Could you check a few things on this model? Use its own coordinates, in mm. A direction names the side the tool comes from. Coordinates: 2 decimals unless noted, no trailing zeros. Loops run counter-clockwise (first coordinate to the right, second up) from the corner with the lowest first, then second, coordinate; pieces in that order, holes last.
1) If I drill on line 1 along Y through (x, z) = (40, -0.25) (3 decimals); line 2 along Y through (x, z) = (50.8, -11.25), over which ranges is the centre line in solid material (lowest first)?
2) Imagine slicing it at A-A on y = 0. Please give me the cut outline in (x, z) (1 decimal).
3) For faces 4 (the face through (-1, 9.525, 0)), 5 (the face through (-1, 0, 12.7)), which set-ups out of +Z, -Z, +X, -X, +Y, -Y let a thin tool reach every point of the face, with its end or its side?
4) Imagine slicing it at C-C on x = -50.8. Please give me the cut outline in (y, z) (1 decimal).
5) Imagine slicing it at B-B on z = 0. Please give me the cut outline in (x, y) (1 decimal), plus the area to 3 significant figures.
6) Thinking about a two-plate mould opening in Y: for faces 1 (the face through (-1, -12.7, 0)), 2 (the face through (-1, 12.7, 0)), 3 (the face through (-1, 0, -9.525)), which applies, released by +Y, released by -Y, zero draft, split by the parting line, or undercut?
7) Imagine slicing it at D-D on x = -33.5. Please give me the cut outline in (y, z) (3 decimals).
Autodesk Inventor part; units mm, degrees
ref_plane "YZ Plane" through (0, 0, 0) normal (1, 0, 0) x (0, 1, 0)
ref_plane "XZ Plane" through (0, 0, 0) normal (0, 1, 0) x (-1, 0, 0)
ref_plane "XY Plane" through (0, 0, 0) normal (0, 0, 1) x (1, 0, 0)
sketch "Sketch1" plane through (0, 0, 0) normal (1, 0, 0) x (0, 1, 0)
  line L0 (-17.78, 0) -> (17.78, 0) construction
  line L1 (0, -17.78) -> (0, 17.78) construction
  line L2 (9.525, 9.525) -> (-9.525, 9.525)
  line L3 (-9.525, 9.525) -> (-9.525, -9.525)
  line L4 (-9.525, -9.525) -> (9.525, -9.525)
  line L5 (9.525, -9.525) -> (9.525, 9.525)
  line L6 (12.7, 12.7) -> (-12.7, 12.7)
  line L7 (-12.7, 12.7) -> (-12.7, -12.7)
  line L8 (-12.7, -12.7) -> (12.7, -12.7)
  line L9 (12.7, -12.7) -> (12.7, 12.7)
  point P0 (0, 0)
  point P1 (0, 12.7)
  point P2 (0, 9.525)
  point P3 (12.7, 0)
  point P4 (9.525, 0)
  dimension "d0" = 3.175
  dimension "d1" = 25.4
extrude "Extrusion1" add sketch "Sketch1" along normal mid plane 127
sketch "Sketch2" plane through (-63.5, -12.7, 12.7) normal (0, 0, 1) x (1, 0, 0)
  line L0 (63.5, -5.08) -> (63.5, 30.48) construction
  line L1 (-29.5275, 12.7) -> (177.165, 12.7) construction
  circle A0 centre (114.3, 12.7) radius 7.9375
  line L2 (127, 25.4) -> (127, 0) construction
  point P0 (63.5, 12.7)
  dimension "d4" = 15.875
  dimension "d5" = 12.7
extrude "Extrusion2" cut sketch "Sketch2" against normal through all
sketch "Sketch3" plane through (-63.5, 12.7, 12.7) normal (0, 1, 0) x (1, 0, 0)
  line L0 (63.5, 30.48) -> (63.5, -5.08) construction
  line L1 (-25.4, 12.7) -> (152.4, 12.7) construction
  circle A0 centre (12.7, 12.7) radius 7.9375
  line L2 (0, 0) -> (0, 25.4) construction
  point P0 (63.5, 12.7)
  dimension "d8" = 12.7
  dimension "d9" = 15.875
extrude "Extrusion3" cut sketch "Sketch3" against normal through all
properties part number "Coupler" material "Aluminum 6061"
Filled in:
1. line 1: y = -12.7 to -9.525, 9.525 to 12.7
1. line 2: y = -12.7 to -7.94, 7.94 to 12.7
2. outline: (-63.5, -12.7) - (42.9, -12.7) - (42.9, -9.5) - (-63.5, -9.5) - close; (-63.5, 9.5) - (42.9, 9.5) - (42.9, 12.7) - (-63.5, 12.7) - close; (58.7, -12.7) - (63.5, -12.7) - (63.5, -9.5) - (58.7, -9.5) - close; (58.7, 9.5) - (63.5, 9.5) - (63.5, 12.7) - (58.7, 12.7) - close
3. face 4: +X, -X
3. face 5: +Z, +X, -X, +Y, -Y
4. outline: (-12.7, -12.7) - (12.7, -12.7) - (12.7, -7.9) - (9.5, -7.9) - (9.5, -9.5) - (-9.5, -9.5) - (-9.5, -7.9) - (-12.7, -7.9) - close; (-12.7, 7.9) - (-9.5, 7.9) - (-9.5, 9.5) - (9.5, 9.5) - (9.5, 7.9) - (12.7, 7.9) - (12.7, 12.7) - (-12.7, 12.7) - close
5. outline: (-63.5, -12.7) - (-58.7, -12.7) - (-58.7, -9.5) - (-63.5, -9.5) - close; (-63.5, 9.5) - (-58.7, 9.5) - (-58.7, 12.7) - (-63.5, 12.7) - close; (-42.9, -12.7) - (63.5, -12.7) - (63.5, -9.5) - (-42.9, -9.5) - close; (-42.9, 9.5) - (63.5, 9.5) - (63.5, 12.7) - (-42.9, 12.7) - close
5. area: 706 mm2
6. face 1: released by -Y
6. face 2: released by +Y
6. face 3: undercut
7. outline: (-12.7, -12.7) - (12.7, -12.7) - (12.7, 12.7) - (-12.7, 12.7) - close; hole (-9.525, -9.525) - (9.525, -9.525) - (9.525, 9.525) - (-9.525, 9.525) - close
